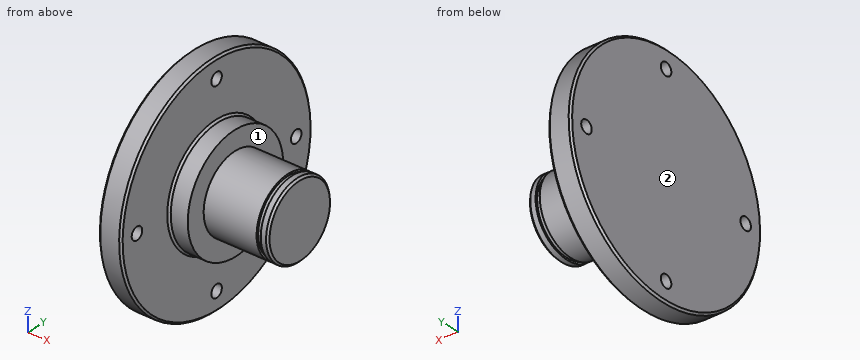
from build123d import *

# Parameters (mm, degrees)
HOLE_WIZARD_M4_1_D = 3.3
CHAMFER_1_SIZE     = 0.5
SKETCH_4_W         = 1.1
SKETCH_4_H         = 0.904012781


with BuildPart() as part:
    # 草图1 → 旋转1 (revolve)
    with BuildSketch(Plane.XY, mode=Mode.PRIVATE) as revolve_1_sk:
        Polygon((0, 0), (0, 30), (6, 30), (6, 15), (11, 15), (11, 10), (28, 10), (28, 0), align=None)
    revolve(revolve_1_sk.sketch.rotate(Axis((-37.713688213, 0, 0), (1, 0, 0)), 90), axis=Axis((-37.713688213, 0, 0), (1, 0, 0)))

    # M4 螺纹孔1 (through all)
    with Locations(Plane(origin=(0, 0, -25), x_dir=(0, 0, -1), z_dir=(-1, 0, 0))):
        with Locations((0, 0), (-25, -25), (-50, 0), (-25, 25)):
            Hole(HOLE_WIZARD_M4_1_D / 2)

    # 倒角1
    chamfer_1_edges = [part.edges().sort_by_distance(p)[0] for p in [
        (28, 0, -10),
        (6, 0, -15),
        (6, 0, -30),
        (0, 0, -30),
    ]]
    chamfer(chamfer_1_edges, length=CHAMFER_1_SIZE)

    # 草图4 → 切除-旋转1 (revolve, cut)
    with BuildSketch(Plane.XY, mode=Mode.PRIVATE) as cut_revolve_1_sk:
        with Locations((25.55, 9.95200639)):
            Rectangle(SKETCH_4_W, SKETCH_4_H)
    revolve(cut_revolve_1_sk.sketch.rotate(Axis((-5.373474488, 0, 0), (1, 0, 0)), 90), axis=Axis((-5.373474488, 0, 0), (1, 0, 0)), mode=Mode.SUBTRACT)


solid = part.part
For this review, take the finished solid that the model builds, in its own axes (mm). Face numbers are marked on the shaded views. A direction names the side the tool comes from. Coordinates: 2 decimals unless noted, no trailing zeros. Loops run counter-clockwise (first coordinate to the right, second up) from the corner with the lowest first, then second, coordinate; pieces in that order, holes last. Notation, with made-up numbers: (84.5, -17) - (118.5, -17) arc R14 cw to (118.5, 1) - close; hole circle Ø10 at (-2, 46.25). An arc over 180 degrees is marked (long way). Use a Markdown table: item, result. Add a question column.
Item 1: For line 1 (Y direction, x = 3.7, z = 0); line 2 (X direction, y = 11.5, z = -18); line 3 (Z direction, x = 5.25, y = 26.5), list the stretches that pass through material, from the lowest coordinate up.
Item 2: We need section C-C (x = 16.75). Give the boundary of the cut face in (y, z).
Item 3: Tool access review of the marked faces 1 and 2: name each direction out of +Z, -Z, +X, -X, +Y, -Y from which nothing blocks a thin tool from reaching the whole face with its end or side.
Item 4: We need section D-D (x = 9). Give the boundary of the cut face in (y, z).
Item 5: We need section A-A (x = 4.5). Give the boundary of the cut face in (y, z), and give its area (3 significant figures).
Item 6: Insertion check: pin 1 Ø4.5 at (y, z) = (-25, 0) entering from +X; pin 2 Ø1 at (x, z) = (5.5, 9) entering from -Y; pin 3 Ø2.5 at (y, z) = (0, 25) entering from -X; pin 4 Ø10 at (x, y) = (4, 17) entering from +Z. Each pin has a flat end and moves straight along its axis. Give the tip position at first contact, or say it passes through.
Item 7: We need section B-B (z = 0). Give the number of separate pieces and of enclosed holes in the cut face, and give its area (3 significant figures).
Results list:
| question | item | result |
|---|---|---|
| 1 | line 1 | y = -30 to -26.65, -23.35 to 23.35, 26.65 to 30 |
| 1 | line 2 | x = 0 to 6 |
| 1 | line 3 | z = -14.06 to -0.69, 0.69 to 14.06 |
| 2 | outline | circle Ø20 at (0, 0) |
| 3 | face 1 | +X |
| 3 | face 2 | +Z, -Z, -X, +Y, -Y |
| 4 | outline | circle Ø30 at (0, 0) |
| 5 | outline | circle Ø60 at (0, 0); hole circle Ø3.3 at (-25, 0); hole circle Ø3.3 at (0, -25); hole circle Ø3.3 at (0, 25); hole circle Ø3.3 at (25, 0) |
| 5 | area | 2,790 mm^2 |
| 6 | pin 1 | stops at x = 6 |
| 6 | pin 2 | stops at y = -28.77 |
| 6 | pin 3 | passes through |
| 6 | pin 4 | stops at z = 27.5 |
| 7 | separate pieces | 3 |
| 7 | enclosed holes | 0 |
| 7 | area | 809 mm^2 |
